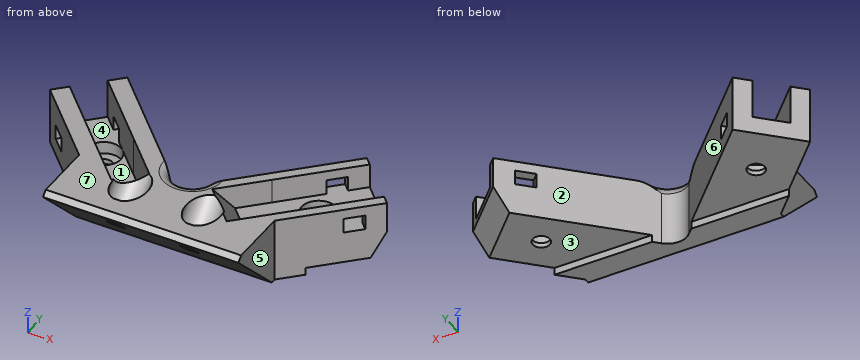
```python
from build123d import *

# Parameters (mm, degrees)
BOSS_EXTRU_1_DEPTH       = 15
ENL_V_MAT_EXTRU_1_DEPTH  = 5
ENL_V_MAT_EXTRU_2_DEPTH  = 8
CHANFREIN1_SIZE          = 11
CHANFREIN1_SIZE_2        = 13.109289519
ESQUISSE8_W              = 3
ESQUISSE8_H              = 4
ENL_V_MAT_EXTRU_6_DEPTH  = 50
ESQUISSE7_W              = 4
ESQUISSE7_H              = 3
ENL_V_MAT_EXTRU_5_DEPTH  = 50
ESQUISSE6_W              = 69.009802941
ESQUISSE6_H              = 2
ENL_V_MAT_EXTRU_4_DEPTH  = 100
CHANFREIN2_SIZE          = 11
CHANFREIN2_SIZE_2        = 30.222251614
ESQUISSE9_W              = 40
ESQUISSE9_H              = 13
BOSS_EXTRU_2_DEPTH       = 5
CHANFREIN4_SIZE          = 12
ESQUISSE10_R             = 1.75
ENL_V_MAT_EXTRU_7_DEPTH  = 1.5
CHANFREIN5_SIZE          = 3
CHANFREIN5_SIZE2         = 5.196152423
ESQUISSE11_R             = 1.75
ENL_V_MAT_EXTRU_8_DEPTH  = 50.355263045
ESQUISSE12_R             = 3.5
ENL_V_MAT_EXTRU_9_DEPTH  = 2.5
ESQUISSE13_R             = 3.5
ENL_V_MAT_EXTRU_10_DEPTH = 5.5
CONG_1_R                 = 4
CHANFREIN10_SIZE         = 1
ESQUISSE14_R             = 1.85
ENL_V_MAT_EXTRU_11_DEPTH = 46.879646797
ENL_V_START              = -4
ESQUISSE15_R             = 3.5
ENL_V_MAT_EXTRU_12_DEPTH = 42.879646797


with BuildPart() as part:
    # Esquisse1 → Boss.-Extru.1 (new body)
    with BuildSketch(Plane.XY):
        Polygon((-20, 0), (20, 0), (20, 8), (34.7949995, 22.5020002), (24.9949995, 32.5), (0, 8), (-24.014803441, 32.5), (-34.214803441, 22.5020002), (-20, 8), align=None)
    extrude(amount=BOSS_EXTRU_1_DEPTH)

    # Esquisse2 → Enlèv. mat.-Extru.1 (cut)
    with BuildSketch(Plane.XY.offset(15)):
        Polygon((26.3949995, 31.071714314), (13.540428329, 18.471714314), (20.540428329, 11.330285886), (33.3949995, 23.930285886), align=None)
    extrude(amount=-ENL_V_MAT_EXTRU_1_DEPTH, mode=Mode.SUBTRACT)

    # Esquisse3 → Enlèv. mat.-Extru.2 (cut)
    with BuildSketch(Plane.XY.offset(15)):
        Polygon((-31.614303391, 25.0510001), (-19.014303391, 12.196428929), (-14.015303491, 17.096428929), (-26.615303491, 29.9510001), align=None)
    extrude(amount=-ENL_V_MAT_EXTRU_2_DEPTH, mode=Mode.SUBTRACT)

    # Chanfrein1
    # the kernel refuses this chamfer: 13.109289519, 11 mm, written as the material it takes off along each edge
    with BuildSketch(Plane(origin=(13.540428329, 18.471714314, 15), x_dir=(-0.7141428428542841, -0.7000000000000011, 0), z_dir=(0.7000000000000011, -0.7141428428542841, 0))) as chanfrein1_piece_1_section:
        Polygon((CHANFREIN1_SIZE, 0), (0, CHANFREIN1_SIZE_2), (0, 0), align=None)
    chanfrein1_piece_1 = extrude(amount=10, mode=Mode.PRIVATE)
    chanfrein1_piece_1 = split(chanfrein1_piece_1, bisect_by=Plane(origin=(13.540428329, 18.471714314, 10), z_dir=(0, 0, 1)), keep=Keep.TOP, mode=Mode.PRIVATE)
    add(chanfrein1_piece_1, mode=Mode.SUBTRACT)

    # Esquisse8 → Enlèv. mat.-Extru.6 (cut)
    with BuildSketch(Plane(origin=(-6.20080008, -6.0779998, 0), x_dir=(0, 0, 1), z_dir=(-0.7141428428542848, -0.7000000000000004, 0))):
        with Locations((8.5, 34.020004802)):
            Rectangle(ESQUISSE8_W, ESQUISSE8_H)
    extrude(amount=-ENL_V_MAT_EXTRU_6_DEPTH, mode=Mode.SUBTRACT)

    # Esquisse7 → Enlèv. mat.-Extru.5 (cut)
    with BuildSketch(Plane(origin=(5.80080008, -5.9179998, 0), x_dir=(0.714142842854285, 0.7000000000000002, 0), z_dir=(0.7000000000000002, -0.714142842854285, 0))):
        with Locations((34.6, 11.5)):
            Rectangle(ESQUISSE7_W, ESQUISSE7_H)
    extrude(amount=-ENL_V_MAT_EXTRU_5_DEPTH, mode=Mode.SUBTRACT)

    # Esquisse6 → Enlèv. mat.-Extru.4 (cut)
    with BuildSketch(Plane.XZ):
        with Locations((0.29009803, 1)):
            Rectangle(ESQUISSE6_W, ESQUISSE6_H)
    extrude(amount=-ENL_V_MAT_EXTRU_4_DEPTH, mode=Mode.SUBTRACT)

    # Chanfrein2
    # the kernel refuses this chamfer: 30.222251614, 11 mm, written as the material it takes off along each edge
    with BuildSketch(Plane(origin=(-19.014303391, 12.196428929, 15), x_dir=(0.7000000000000006, -0.7141428428542845, 0), z_dir=(0.7141428428542845, 0.7000000000000005, 0))) as chanfrein2_piece_1_section:
        Polygon((CHANFREIN2_SIZE, 0), (0, CHANFREIN2_SIZE_2), (0, 0), align=None)
    chanfrein2_piece_1 = extrude(amount=7, mode=Mode.PRIVATE)
    chanfrein2_piece_1 = split(chanfrein2_piece_1, bisect_by=Plane(origin=(-19.014303391, 12.196428929, 7), z_dir=(0, 0, 1)), keep=Keep.TOP, mode=Mode.PRIVATE)
    add(chanfrein2_piece_1, mode=Mode.SUBTRACT)

    # Esquisse9 → Boss.-Extru.2 (add)
    with BuildSketch(Plane.XZ):
        with Locations((0, 8.5)):
            Rectangle(ESQUISSE9_W, ESQUISSE9_H)
    extrude(amount=BOSS_EXTRU_2_DEPTH)

    # Chanfrein4
    chanfrein4_edges = [part.edges().sort_by_distance(p)[0] for p in [
        (0, -5, 2),
    ]]
    chamfer(chanfrein4_edges, length=CHANFREIN4_SIZE)

    # Esquisse10 → Enlèv. mat.-Extru.7 (cut)
    with BuildSketch(Plane(origin=(0, 0, 2), x_dir=(-1, 0, 0), z_dir=(0, 0, -1))):
        Polygon((-35.24, 27.99759976), (-35.24, 11.99759976), (34.76, 11.99759976), (34.76, 27.99759976), (34.76, 37.99759976), (-35.24, 37.99759976), align=None)
        with Locations((-22.24, 19.99759976)):
            Circle(ESQUISSE10_R, mode=Mode.SUBTRACT)
        with Locations((21.76, 19.99759976)):
            Circle(ESQUISSE10_R, mode=Mode.SUBTRACT)
    extrude(amount=-ENL_V_MAT_EXTRU_7_DEPTH, mode=Mode.SUBTRACT)

    # Chanfrein5
    chanfrein5_edges = [part.edges().sort_by_distance(p)[0] for p in [
        (29.8949995, 27.5010001, 3.5),
    ]]
    chanfrein5_side = [part.faces().sort_by_distance(p)[0] for p in [
        (29.178170188, 17.513536316, 3.5),
    ]]
    chamfer(chanfrein5_edges, length=CHANFREIN5_SIZE, length2=CHANFREIN5_SIZE2, reference=chanfrein5_side[0])

    # Esquisse11 → Enlèv. mat.-Extru.8 (cut, through all)
    with BuildSketch(Plane(origin=(0, 0, 2), x_dir=(-1, 0, 0), z_dir=(0, 0, -1))):
        with Locations((-22.24, 19.99759976)):
            Circle(ESQUISSE11_R)
        with Locations((21.76, 19.99759976)):
            Circle(ESQUISSE11_R)
    extrude(amount=-ENL_V_MAT_EXTRU_8_DEPTH, mode=Mode.SUBTRACT)

    # Esquisse12 → Enlèv. mat.-Extru.9 (cut)
    with BuildSketch(Plane.XY.offset(7)):
        with Locations((-21.76, 19.99759976)):
            Circle(ESQUISSE12_R)
    extrude(amount=-ENL_V_MAT_EXTRU_9_DEPTH, mode=Mode.SUBTRACT)

    # Esquisse13 → Enlèv. mat.-Extru.10 (cut)
    with BuildSketch(Plane.XY.offset(10)):
        with Locations((22.24, 19.99759976)):
            Circle(ESQUISSE13_R)
    extrude(amount=-ENL_V_MAT_EXTRU_10_DEPTH, mode=Mode.SUBTRACT)

    # Congé1
    cong_1_edges = [part.edges().sort_by_distance(p)[0] for p in [
        (0, 8, 8.5),
    ]]
    fillet(cong_1_edges, radius=CONG_1_R)

    # Chanfrein10
    chanfrein10_edges = [part.edges().sort_by_distance(p)[0] for p in [
        (0, -5, 15),
    ]]
    chamfer(chanfrein10_edges, length=CHANFREIN10_SIZE - 0.0001)  # a hair under: the kernel refuses the full size

    # Esquisse14 → Enlèv. mat.-Extru.11 (cut, through all)
    with BuildSketch(Plane(origin=(0, 4.5, 4.5), x_dir=(1, 0, 0), z_dir=(0, -0.7071067811865464, -0.7071067811865488))):
        with Locations(Location((-7.5, 7.435028843, 0), (0, 0, 270))):
            Circle(ESQUISSE14_R)
        with Locations(Location((7.5, 7.435028843, 0), (0, 0, 270))):
            Circle(ESQUISSE14_R)
    extrude(amount=-ENL_V_MAT_EXTRU_11_DEPTH, mode=Mode.SUBTRACT)

    # Esquisse15 → Enlèv. mat.-Extru.12 (cut, through all)
    with BuildSketch(Plane(origin=(0, 4.5, 4.5), x_dir=(1, 0, 0), z_dir=(0, -0.7071067811865464, -0.7071067811865488)).offset(ENL_V_START)):
        with Locations((-7.5, 7.435028843)):
            Circle(ESQUISSE15_R)
        with Locations((7.5, 7.435028843)):
            Circle(ESQUISSE15_R)
    extrude(amount=-ENL_V_MAT_EXTRU_12_DEPTH, mode=Mode.SUBTRACT)

    # Congé2: read off the stored shape, not the designer's step
    # Congé2 outline → Congé2 (revolve, cut)
    with BuildSketch(Plane(origin=(0.056571371, 13.656571371, 0), x_dir=(1, 0, 0), z_dir=(0, -1, 0))):
        with BuildLine():
            ThreePointArc((4, 13), (4.585786438, 14.414213562), (6, 15))
            Line((6, 15), (4, 15))
            Line((4, 15), (4, 13))
        make_face()
    revolve(axis=Axis((0.056571371, 13.656571371, 0), (0, 0, 1)), mode=Mode.SUBTRACT)


solid = part.part
```
The model under review builds one solid part; all positions refer to its coordinate system, in mm. Face numbers are marked on the shaded views. A direction names the side the tool comes from. Round coordinates to 2 decimals unless told otherwise and drop trailing zeros. Answer as a JSON object with one key per item and string values.
(1) Tool access review of the marked faces 1, 2, 3 and 4: name each direction out of +Z, -Z, +X, -X, +Y, -Y from which nothing blocks a thin tool from reaching the whole face with its end or side.
Resolved:
{"face 1": "+Z", "face 2": "+Z, -Z, +Y", "face 3": "-Z, +X, -X, +Y", "face 4": "none"}
(2) Draft analysis for pull direction X (two halves, no side actions). For the marked faces 5, 6 and 7, state which applies: released by +X, released by -X, zero draft, split by the parting line, or undercut.
Resolved:
{"face 5": "released by +X", "face 6": "undercut", "face 7": "zero draft"}
(3) Clearance check with flat-ended pins moving along their axes: P1, Ø5, axis at x = 20.5, z = 7.5, coming from the -Y side; P2, Ø4, axis at y = 17, z = 7.5, coming from the +X side; P3, Ø6.5, axis at x = -21.76, y = 20, coming from the +Z side. State where each tip first meets the part, or that it passes through.
Resolved:
{"P1": "y = -0.95", "P2": "x = 31.22", "P3": "z = 4.5"}
(4) To check wall thickness, follow line 1 along X through (y, z) = (23, 8.75); line 2 along X through (y, z) = (17, 7.5); line 3 along Z through (x, y) = (20.5, 17). State the ranges of each line that lie inside material, in increasing order.
Resolved:
{"line 1": "-33.71 to -29.6, -19.8 to -14.7, 15.3 to 20.44, 24.04 to 34.31", "line 2": "-28.4 to -23.72, -13.92 to -8.82, 9.18 to 20.43, 24.05 to 29.18", "line 3": "3.5 to 4.5"}
